from build123d import *

# Parameters (mm, degrees)
IZIM1_W                     = 90
IZIM1_H                     = 60
Y_KSEKLIK_EKSTR_ZYON1_DEPTH = 3
IZIM2_W                     = 96
IZIM2_H                     = 66
IZIM2_W_2                   = 90
IZIM2_H_2                   = 60
Y_KSEKLIK_EKSTR_ZYON2_DEPTH = 38
IZIM3_W                     = 60
IZIM3_H                     = 3
KES_EKSTR_ZYON1_DEPTH       = 35
IZIM4_W                     = 66
IZIM4_H                     = 96
Y_KSEKLIK_EKSTR_ZYON3_DEPTH = 3
RADYUS4_R                   = 3
RADYUS5_R                   = 3
RADYUS6_R                   = 3
RADYUS7_R                   = 3


with BuildPart() as part:
    # Çizim1 → Yükseklik-Ekstrüzyon1 (new body)
    with BuildSketch(Plane(origin=(0, 0, 0), x_dir=(0, 1, 0), z_dir=(0, 0, 1))):
        with Locations((45, -30)):
            Rectangle(IZIM1_W, IZIM1_H)
    extrude(amount=Y_KSEKLIK_EKSTR_ZYON1_DEPTH)

    # Çizim2 → Yükseklik-Ekstrüzyon2 (add)
    with BuildSketch(Plane(origin=(0, 0, 0), x_dir=(0, 1, 0), z_dir=(0, 0, 1))):
        with Locations((45, -30)):
            Rectangle(IZIM2_W, IZIM2_H)
        with Locations((45, -30)):
            Rectangle(IZIM2_W_2, IZIM2_H_2, mode=Mode.SUBTRACT)
    extrude(amount=Y_KSEKLIK_EKSTR_ZYON2_DEPTH)

    # Çizim3 → Kes-Ekstrüzyon1 (cut)
    with BuildSketch(Plane.XY.offset(38)):
        with Locations((30, 91.5)):
            Rectangle(IZIM3_W, IZIM3_H)
    extrude(amount=-KES_EKSTR_ZYON1_DEPTH, mode=Mode.SUBTRACT)

    # Çizim4 → Yükseklik-Ekstrüzyon3 (add)
    with BuildSketch(Plane.XY.offset(38)):
        with Locations((30, 45)):
            Rectangle(IZIM4_W, IZIM4_H)
    extrude(amount=Y_KSEKLIK_EKSTR_ZYON3_DEPTH)

    # Radyus4
    radyus4_edges = [part.edges().sort_by_distance(p)[0] for p in [
        (-3, -3, 20.5),
    ]]
    fillet(radyus4_edges, radius=RADYUS4_R)

    # Radyus5
    radyus5_edges = [part.edges().sort_by_distance(p)[0] for p in [
        (63, -3, 20.5),
    ]]
    fillet(radyus5_edges, radius=RADYUS5_R)

    # Radyus6
    radyus6_edges = [part.edges().sort_by_distance(p)[0] for p in [
        (-3, 46.5, 41),
        (30, -3, 41),
        (-2.121320344, -2.121320344, 41),
        (63, 46.5, 41),
        (62.121320344, -2.121320344, 41),
    ]]
    fillet(radyus6_edges, radius=RADYUS6_R)

    # Radyus7
    radyus7_edges = [part.edges().sort_by_distance(p)[0] for p in [
        (-3, 46.5, 0),
        (30, -3, 0),
        (-2.121320344, -2.121320344, 0),
        (63, 46.5, 0),
        (62.121320344, -2.121320344, 0),
    ]]
    fillet(radyus7_edges, radius=RADYUS7_R)


solid = part.part
Check sheet for the modelled part. Datum: model origin and axes. Units: mm. A direction names the side the tool comes from. Give positions to 0.01 mm unless a question says otherwise; leave off trailing zeros. Write each loop counter-clockwise with the first axis right and the second up, starting at its lowest first coordinate (ties: lowest second). Pieces come first, ordered by that corner, then holes. Notation, with made-up numbers: (25.25, 75) -> (71.25, 75) arc R19 ccw to (71.25, 109) -> close; hole circle Ø3 at (11, 41.25). An arc over 180 degrees is marked (long way). Use one line per item in the form item = value. Start each with the question number.
1. Section check C-C (x = 54.5). Record the cut outline in (y, z), and give its area (3 significant figures).
2. Go/stop test with a flat-tipped pin: P1, Ø17.5, axis at x = 24, z = 19.5, coming from the +Y side. Record where the tip stops, or that it passes through.
3. Section check A-A (y = 54). Record the cut outline in (x, z).
4. Mould release check, pull along X, two halves, no side actions. Record for faces 1 (the flat face through (60, 46, 20)), 2 (the flat face through (-3, 46, 20)), 3 (the flat face through (30, 47, 41)): pulls with the +X half, pulls with the -X half, needs draft (parallel to the pull), parting line crosses it, or undercut.
5. Thickness scan on line 1 along X through (y, z) = (86, 32.5); line 2 along Z through (x, y) = (38, 68); line 3 along Y through (x, z) = (12, 30.5). Record the ranges inside material, lowest first. Write a range as from..to.
6. Access from +Z, -Z, +X, -X, +Y, -Y to the whole of each face (thin tool, end or side, straight path). Record for faces 4 (the cylindrical face through (-2.14, -2.1, 20.74)), 5 (the flat face through (30, 0, 20)).
7. Section check B-B (z = 16.5). Record the cut outline in (x, y).
Conclusion:
q1.outline = (-3, 3) arc R3 ccw to (0, 0) -> (93, 0) -> (93, 3) -> (0, 3) -> (0, 38) -> (93, 38) -> (93, 41) -> (0, 41) arc R3 ccw to (-3, 38) -> close
q1.area = 677 mm²
q2.P1 = 0
q3.outline = (-3, 3) arc R3 ccw to (0, 0) -> (60, 0) arc R3 ccw to (63, 3) -> (63, 38) arc R3 ccw to (60, 41) -> (0, 41) arc R3 ccw to (-3, 38) -> close; hole (0, 3) -> (60, 3) -> (60, 38) -> (0, 38) -> close
q4.face_1 = undercut
q4.face_2 = pulls with the -X half
q4.face_3 = needs draft
q5.line_1 = -3..0, 60..63
q5.line_2 = 0..3, 38..41
q5.line_3 = -3..0
q6.face_4 = +Z, -Z, -X, -Y
q6.face_5 = +Y
q7.outline = (-3, 0) arc R3 ccw to (0, -3) -> (60, -3) arc R3 ccw to (63, 0) -> (63, 93) -> (60, 93) -> (60, 0) -> (0, 0) -> (0, 93) -> (-3, 93) -> close
